from build123d import *

# Parameters (mm, degrees)
SKETCH1_R           = 1.397
SKETCH1_R_2         = 1.651
SKETCH1_R_3         = 1.016
SKETCH1_W           = 58.544107304
SKETCH1_H           = 8.89
SKETCH1_W_2         = 6.35
SKETCH1_H_2         = 3.175
BOSS_EXTRUDE1_DEPTH = 3.175


with BuildPart() as part:
    # Sketch1 → Boss-Extrude1 (new body)
    with BuildSketch(Plane(origin=(0, 0, 0), x_dir=(1, 0, 0), z_dir=(0, 1, 0))):
        with BuildLine():
            Line((38.407265908, 13.335), (41.582265908, 13.335))
            Line((41.582265908, 13.335), (50.342102347, 13.335))
            ThreePointArc((50.342102347, 13.335), (57.058059725, 24.74076345), (67.270928268, 33.160552015))
            ThreePointArc((67.270928268, 33.160552015), (-10.756431789, 74.224653419), (-73.916912814, 12.7))
            Line((-73.916912814, 12.7), (-73.916912814, -12.7))
            ThreePointArc((-73.916912814, -12.7), (-10.756431789, -74.224653419), (67.270928268, -33.160552015))
            ThreePointArc((67.270928268, -33.160552015), (60.584216496, -28.355013333), (55.086193863, -22.225))
            ThreePointArc((55.086193863, -22.225), (52.41895011, -17.937530518), (50.342102347, -13.335))
            Line((50.342102347, -13.335), (46.281265908, -13.335))
            Line((46.281265908, -13.335), (41.582265908, -13.335))
            Line((41.582265908, -13.335), (41.582265908, -22.86))
            Line((41.582265908, -22.86), (38.407265908, -22.86))
            Line((38.407265908, -22.86), (38.407265908, -13.335))
            Line((38.407265908, -13.335), (-2.486734092, -13.335))
            Line((-2.486734092, -13.335), (-2.486734092, -6.604))
            Line((-2.486734092, -6.604), (-38.046734092, -6.604))
            Line((-38.046734092, -6.604), (-38.046734092, 6.604))
            Line((-38.046734092, 6.604), (-2.486734092, 6.604))
            Line((-2.486734092, 6.604), (-2.486734092, 13.335))
            Line((-2.486734092, 13.335), (38.407265908, 13.335))
        make_face()
        with Locations(Location((-62.486912814, 6.731, 0), (0, 0, 270))):
            Circle(SKETCH1_R, mode=Mode.SUBTRACT)
        with Locations(Location((-62.486912814, -6.731, 0), (0, 0, 270))):
            Circle(SKETCH1_R, mode=Mode.SUBTRACT)
        with Locations(Location((-38.1, -42.418, 0), (0, 0, 270))):
            Circle(SKETCH1_R_2, mode=Mode.SUBTRACT)
        with Locations(Location((38.1, -42.418, 0), (0, 0, 270))):
            Circle(SKETCH1_R_2, mode=Mode.SUBTRACT)
        with Locations(Location((38.1, 42.418, 0), (0, 0, 90))):
            Circle(SKETCH1_R_2, mode=Mode.SUBTRACT)
        with Locations(Location((0, -23.368, 0), (0, 0, 270))):
            Circle(SKETCH1_R_2, mode=Mode.SUBTRACT)
        with Locations(Location((-38.1, 42.418, 0), (0, 0, 90))):
            Circle(SKETCH1_R_2, mode=Mode.SUBTRACT)
        with Locations(Location((0, 23.368, 0), (0, 0, 90))):
            Circle(SKETCH1_R_2, mode=Mode.SUBTRACT)
        with Locations(Location((29.272053652, -37.649461806, 0), (0, 0, 270))):
            Circle(SKETCH1_R, mode=Mode.SUBTRACT)
        with Locations(Location((-58.676912814, 34.29, 0), (0, 0, 270))):
            Circle(SKETCH1_R_2, mode=Mode.SUBTRACT)
        with Locations(Location((62.141053559, -35.830642926, 0), (0, 0, 270))):
            Circle(SKETCH1_R_3, mode=Mode.SUBTRACT)
        with Locations(Location((56.570777105, -32.679132142, 0), (0, 0, 270))):
            Circle(SKETCH1_R_3, mode=Mode.SUBTRACT)
        with Locations(Location((-58.676912814, -34.29, 0), (0, 0, 270))):
            Circle(SKETCH1_R_2, mode=Mode.SUBTRACT)
        with Locations(Location((29.272053652, -24.187461806, 0), (0, 0, 270))):
            Circle(SKETCH1_R, mode=Mode.SUBTRACT)
        with Locations(Location((29.272053652, 37.649461806, 0), (0, 0, 90))):
            Circle(SKETCH1_R, mode=Mode.SUBTRACT)
        with Locations(Location((29.272053652, 24.187461806, 0), (0, 0, 90))):
            Circle(SKETCH1_R, mode=Mode.SUBTRACT)
        with Locations(Location((8.99925, -43.353461806, 0), (0, 0, 270))):
            Circle(SKETCH1_R_2, mode=Mode.SUBTRACT)
        with Locations(Location((-9.00075, -43.353461806, 0), (0, 0, 270))):
            Circle(SKETCH1_R_2, mode=Mode.SUBTRACT)
        with Locations(Location((-9.00075, 43.353461806, 0), (0, 0, 90))):
            Circle(SKETCH1_R_2, mode=Mode.SUBTRACT)
        with Locations(Location((8.99925, 43.353461806, 0), (0, 0, 90))):
            Circle(SKETCH1_R_2, mode=Mode.SUBTRACT)
        with Locations(Location((62.141053559, 35.830642926, 0), (0, 0, 270))):
            Circle(SKETCH1_R_3, mode=Mode.SUBTRACT)
        with Locations(Location((56.570777105, 32.679132142, 0), (0, 0, 270))):
            Circle(SKETCH1_R_3, mode=Mode.SUBTRACT)
        with Locations(Location((22.278265908, 19.05, 0), (0, 0, 270))):
            Circle(SKETCH1_R_2, mode=Mode.SUBTRACT)
        with Locations(Location((22.278265908, -19.05, 0), (0, 0, 270))):
            Circle(SKETCH1_R_2, mode=Mode.SUBTRACT)
        with Locations(Location((-22.171734092, -19.05, 0), (0, 0, 270))):
            Circle(SKETCH1_R_2, mode=Mode.SUBTRACT)
        with Locations(Location((-22.171734092, 19.05, 0), (0, 0, 270))):
            Circle(SKETCH1_R_2, mode=Mode.SUBTRACT)
        with Locations((0, -61.144461806)):
            Rectangle(SKETCH1_W, SKETCH1_H, mode=Mode.SUBTRACT)
        with Locations((0, 61.144461806)):
            Rectangle(SKETCH1_W, SKETCH1_H, mode=Mode.SUBTRACT)
        with Locations((55.791053559, -40.593142926)):
            Rectangle(SKETCH1_W_2, SKETCH1_H_2, mode=Mode.SUBTRACT)
        with Locations((55.791053559, 40.593142926)):
            Rectangle(SKETCH1_W_2, SKETCH1_H_2, mode=Mode.SUBTRACT)
        Polygon((32.44100721, -56.895314679), (35.719111901, -62.333745485), (38.438327304, -60.694693139), (35.160222613, -55.256262334), align=None, mode=Mode.SUBTRACT)
        Polygon((-32.44100721, -56.895314679), (-35.160222613, -55.256262334), (-38.438327304, -60.694693139), (-35.719111901, -62.333745485), align=None, mode=Mode.SUBTRACT)
        Polygon((-35.160222613, 55.256262334), (-38.438327304, 60.694693139), (-35.719111901, 62.333745485), (-32.44100721, 56.895314679), align=None, mode=Mode.SUBTRACT)
        Polygon((35.160222613, 55.256262334), (38.438327304, 60.694693139), (35.719111901, 62.333745485), (32.44100721, 56.895314679), align=None, mode=Mode.SUBTRACT)
        with Locations((-67.566912814, 0)):
            Rectangle(SKETCH1_W_2, SKETCH1_H_2, mode=Mode.SUBTRACT)
    extrude(amount=BOSS_EXTRUDE1_DEPTH)


solid = part.part
The model under review builds one solid part; all positions refer to its coordinate system, in mm. A direction names the side the tool comes from. Coordinates: 2 decimals unless noted, no trailing zeros. Write each loop counter-clockwise with the first axis right and the second up, starting at its lowest first coordinate (ties: lowest second). Pieces come first, ordered by that corner, then holes. Notation, with made-up numbers: (56, 37) - (107, 37) arc R11 cw to (107, 54) - close; hole circle Ø2 at (5, -33). An arc over 180 degrees is marked (long way). Answer as a JSON object with one key per item and string values. Group by question number.
1. Machinability: for faces 1 (the face through (-4, 3.175, 16)), 2 (the face through (-68, 2, -1.588)), 3 (the face through (-38.047, 2, 0)), which of the approach directions +Z, -Z, +X, -X, +Y, -Y give a long, thin tool a straight path to every point of the face, cutting with its end or side? Answer none if there is none.
2. Add section B-B (x = 44). Give the boundary of the cut face in (y, z) (3 decimals), plus the area to 3 significant figures.
3. Add section C-C (z = -19.05). Give the boundary of the cut face in (x, y) (3 decimals).
4. Add section A-A (z = 19.05). Give the boundary of the cut face in (x, y) (3 decimals), plus the area to 3 significant figures.
5. Add section D-D (y = 2.3). Give the number of separate pieces and of enclosed holes in the cut face, plus the area to 3 significant figures.
6. Mouldability with a two-part tool opening along X and no side actions: class faces 4 (the face through (-2.487, 2, -10)), 5 (the face through (-8.928, 1.565, 41.704)), 6 (the face through (-12.061, 1.565, 74.024)), 7 (the face through (46, 2, 13.335)) as pulls with the +X half, pulls with the -X half, needs draft (parallel to the pull), parting line crosses it, or undercut.
7. To check wall thickness, follow probe 1 along Z at (x, y) = (11.5, 0.4) (3 decimals); probe 2 along X at (y, z) = (1.35, 57.5); probe 3 along Z at (x, y) = (-58.5, 3). State the ranges of each line that lie inside material, in increasing order.
8. Clearance check with flat-ended pins moving along their axes: pin 1 Ø12 at (x, z) = (52.5, 11.5) entering from +Y (3 decimals); pin 2 Ø1.5 at (y, z) = (2.5, -18.5) entering from +X; pin 3 Ø1.6 at (x, y) = (55, 2) entering from +Z; pin 4 Ø1 at (y, z) = (1.5, 10) entering from +X. State where each tip first meets the part, or that it passes through.
Findings:
{
 "1": {"face 1": "+Z, -Z, +X, -X, +Y", "face 2": "+Y, -Y", "face 3": "+X, +Y, -Y"},
 "2": {"outline": "(0, -60.737) - (3.175, -60.737) - (3.175, -13.335) - (0, -13.335) - close; (0, 13.335) - (3.175, 13.335) - (3.175, 60.737) - (0, 60.737) - close", "area": "301 mm²"},
 "3": {"outline": "(-72.54, 0) - (-23.823, 0) - (-23.823, 3.175) - (-72.54, 3.175) - close; (-20.521, 0) - (20.627, 0) - (20.627, 3.175) - (-20.521, 3.175) - close; (23.929, 0) - (53.037, 0) - (53.037, 3.175) - (23.929, 3.175) - close"},
 "4": {"outline": "(-72.54, 0) - (-23.823, 0) - (-23.823, 3.175) - (-72.54, 3.175) - close; (-20.521, 0) - (20.627, 0) - (20.627, 3.175) - (-20.521, 3.175) - close; (23.929, 0) - (38.407, 0) - (38.407, 3.175) - (23.929, 3.175) - close; (41.582, 0) - (53.037, 0) - (53.037, 3.175) - (41.582, 3.175) - close", "area": "368 mm²"},
 "5": {"separate pieces": "1", "enclosed holes": "35", "area": "13,200 mm²"},
 "6": {"face 4": "pulls with the +X half", "face 5": "undercut", "face 6": "parting line crosses it", "face 7": "needs draft"},
 "7": {"probe 1": "-74.113 to -65.589, -56.699 to -13.335, 13.335 to 56.699, 65.589 to 74.113", "probe 2": "-48.15 to -36.51, -32.81 to -29.27, 29.27 to 32.81, 36.51 to 48.15", "probe 3": "-46.93 to -35.93, -32.65 to 32.65, 35.93 to 46.93"},
 "8": {"pin 1": "y = 3.175", "pin 2": "x = 53.15", "pin 3": "z = 51.84", "pin 4": "x = -2.49"}
}
